Here's how the part is built. I have some questions about the finished solid (model axes, mm). A direction names the side the tool comes from. Coordinates: 2 decimals unless noted, no trailing zeros. Write each loop counter-clockwise with the first axis right and the second up, starting at its lowest first coordinate (ties: lowest second). Pieces come first, ordered by that corner, then holes. Notation, with made-up numbers: (31.25, 5) -> (57.25, 5) arc R16 ccw to (57.25, 11) -> close; hole circle Ø2 at (-0.75, -30). An arc over 180 degrees is marked (long way). Put each result on its own line as item: value. Start each with the question number.
Item 1: I want a section at B-B, the plane x = -161.5. List the corners of the cut face in (y, z) for me.
Item 2: I want a section at A-A, the plane z = 301. List the corners of the cut face in (x, y) for me, then the cut area to 3 significant figures.
Item 3: For pin 1 (2 mm diameter, centred on x = -138, y = -9.5, fed in from -Z); pin 2 (10 mm diameter, centred on x = -43.5, y = -9.5, fed in from -Z); pin 3 (12.5 mm diameter, centred on x = -241, y = -6.5, fed in from -Z), each with a flat end and sliding along its axis, tell me the tip position at first contact or that it passes through.
Item 4: I need wall thicknesses on line 1 (X direction, y = -8.5, z = 284); line 2 (Y direction, x = 304.8, z = 744.75); line 3 (X direction, y = -24, z = 362.5). Which ranges of each line are inside material? Lowest first, please. Write a range as [from, to].
Item 5: On a 3-axis mill with a long thin cutter (end or side, diameter ignored), from which of +Z, -Z, +X, -X, +Y, -Y can I reach the whole of each face in a straight line? I mean faces 1 (the face through (172.37, -12.52, 244.8)), 2 (the face through (355.6, -13, 391)), 3 (the face through (381, -13, 376)). Say none if no direction works.
Item 6: I want a section at C-C, the plane z = 603.5. List the corners of the cut face in (x, y) for me, then the cut area to 3 significant figures.
Item 7: If we mould it in two halves opening along Z, with no side actions, what happens to faces 4 (the face through (-75.133, -12.522, 629.898)), 5 (the face through (-177.267, -12.522, 238.038)), 6 (the face through (-381, -13, 386)), 7 (the face through (5, -13, 762))? For each: released by +Z, released by -Z, zero draft, split by the parting line, or undercut.
from build123d import *

# Parameters (mm, degrees)
F1_DEPTH = 25.4
F2_R     = 4.7625
F3_DEPTH = 25.4
F4_R     = 4.7625
F5_DEPTH = 25.4


with BuildPart() as f1:
    # F0 (on Front) → F1 (new body)
    with BuildSketch(Plane.XZ):
        Polygon((381, 762), (-381, 762), (-381, 0), (-349.639734, 0), (0, 482.835824), (349.639734, 0), (381, 0), align=None)
        Polygon((-355.6, 35.07619), (-355.6, 736.6), (-183.760266, 736.6), (-15.680133, 504.48934), align=None, mode=Mode.SUBTRACT)
        Polygon((183.760266, 736.6), (355.6, 736.6), (355.6, 35.07619), (15.680133, 504.48934), align=None, mode=Mode.SUBTRACT)
        Polygon((0, 526.142857), (-152.4, 736.6), (152.4, 736.6), align=None, mode=Mode.SUBTRACT)
    extrude(amount=F1_DEPTH)

    # F2 (on face) → F3 (cut)
    with BuildSketch(Plane.XZ.offset(25.4)):
        with Locations((-279.4, 749.3)):
            Circle(F2_R)
        with Locations((0, 749.3)):
            Circle(F2_R)
        with Locations((279.4, 749.3)):
            Circle(F2_R)
    extrude(amount=-F3_DEPTH, mode=Mode.SUBTRACT)

    # F4 (on face) → F5 (cut)
    with BuildSketch(Plane.XY.offset(762)):
        with Locations((-50.8, -12.7)):
            Circle(F4_R)
        with Locations((50.8, -12.7)):
            Circle(F4_R)
        with Locations((304.8, -12.7)):
            Circle(F4_R)
        with Locations((-304.8, -12.7)):
            Circle(F4_R)
    extrude(amount=-F5_DEPTH, mode=Mode.SUBTRACT)


solid = f1.part
Calculated:
1. outline: (-25.4, 259.81) -> (0, 259.81) -> (0, 303.12) -> (-25.4, 303.12) -> close; (-25.4, 705.86) -> (0, 705.86) -> (0, 762) -> (-25.4, 762) -> close
2. outline: (-381, -25.4) -> (-355.6, -25.4) -> (-355.6, 0) -> (-381, 0) -> close; (-163.03, -25.4) -> (-131.67, -25.4) -> (-131.67, 0) -> (-163.03, 0) -> close; (131.67, -25.4) -> (163.03, -25.4) -> (163.03, 0) -> (131.67, 0) -> close; (355.6, -25.4) -> (381, -25.4) -> (381, 0) -> (355.6, 0) -> close
2. area: 2,880 mm2
3. pin 1: stops at z = 290.88
3. pin 2: stops at z = 415.86
3. pin 3: stops at z = 141.4
4. line 1: x = [-381, -355.6], [-175.34, -143.98], [143.98, 175.34], [355.6, 381]
4. line 2: y = [-25.4, -17.46], [-7.94, 0]
4. line 3: x = [-381, -355.6], [-118.5, -87.14], [87.14, 118.5], [355.6, 381]
5. face 1: -Z, +Y, -Y
5. face 2: +Y, -Y
5. face 3: +Z, -Z, +X, +Y, -Y
6. outline: (-381, -25.4) -> (-355.6, -25.4) -> (-355.6, 0) -> (-381, 0) -> close; (-87.38, -25.4) -> (-56.02, -25.4) -> (-56.02, 0) -> (-87.38, 0) -> close; (56.02, -25.4) -> (87.38, -25.4) -> (87.38, 0) -> (56.02, 0) -> close; (355.6, -25.4) -> (381, -25.4) -> (381, 0) -> (355.6, 0) -> close
6. area: 2,880 mm2
7. face 4: undercut
7. face 5: released by -Z
7. face 6: zero draft
7. face 7: released by +Z
